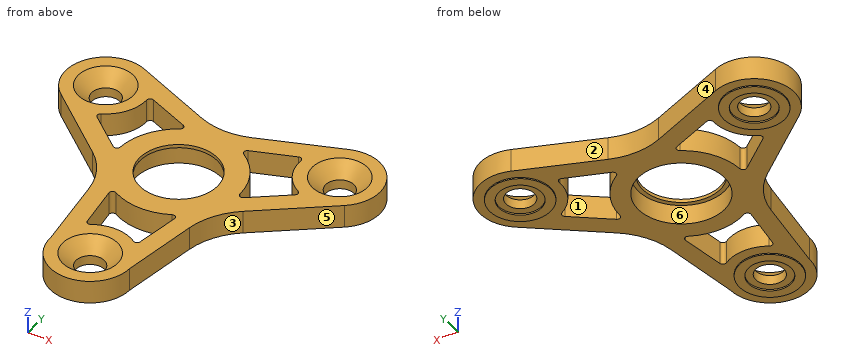
```python
from build123d import *

# Parameters (mm, degrees)
SKETCH_1_R          = 5.935
SKETCH_1_R_2        = 2.095
SKETCH_1_R_3        = 5.74
EXTRUDE_1_DEPTH     = 3.4
SKETCH_3_R          = 6.38
CUT_EXTRUDE_1_DEPTH = 2.9
SKETCH_4_R          = 4.5
EXTRUDE_3_DEPTH     = 0.56
SKETCH_6_R          = 3.15
CUT_EXTRUDE_2_DEPTH = 0.6
SKETCH_7_R          = 3.15
CUT_EXTRUDE_3_DEPTH = 0.6
SKETCH_8_R          = 3.15
CUT_EXTRUDE_4_DEPTH = 0.6
CUT_EXTRUDE_5_DEPTH = 10
SKETCH_13_R         = 4.5
SKETCH_13_R_2       = 3.15
CUT_EXTRUDE_6_DEPTH = 0.37
SKETCH_14_R         = 4.5
SKETCH_14_R_2       = 3.15
CUT_EXTRUDE_7_DEPTH = 0.37
SKETCH_15_R         = 4.5
SKETCH_15_R_2       = 3.15
CUT_EXTRUDE_8_DEPTH = 0.37


with BuildPart() as part:
    # 草图1 → 凸台-拉伸1 (new body)
    # profile 1 of 4: a face of its own
    with BuildSketch(Plane.XY):
        with Locations((-17.593306078, 10.1575)):
            Circle(SKETCH_1_R)
        with Locations((-17.593306078, 10.1575)):
            Circle(SKETCH_1_R_2, mode=Mode.SUBTRACT)
    # profile 2 of 4: a face of its own
    with BuildSketch(Plane.XY):
        with Locations((17.593306078, 10.1575)):
            Circle(SKETCH_1_R)
        with Locations((17.593306078, 10.1575)):
            Circle(SKETCH_1_R_2, mode=Mode.SUBTRACT)
    # profile 3 of 4: a face of its own
    with BuildSketch(Plane.XY):
        with BuildLine():
            Line((-3.823709102, 11.054508427), (-15.39430283, 15.670086481))
            ThreePointArc((-15.39430283, 15.670086481), (-12.680297362, 13.487150186), (-11.658306078, 10.1575))
            ThreePointArc((-11.658306078, 10.1575), (-15.021547784, 4.808641778), (-21.299513922, 5.521958132))
            Line((-21.299513922, 5.521958132), (-11.31029049, -2.464624515))
            ThreePointArc((-11.31029049, -2.464624515), (-8.793601867, -5.406520994), (-7.538053442, -9.068770941))
            Line((-7.538053442, -9.068770941), (-5.935, -20.315))
            ThreePointArc((-5.935, -20.315), (0, -14.38), (5.935, -20.315))
            Line((5.935, -20.315), (7.538053442, -9.068770941))
            ThreePointArc((7.538053442, -9.068770941), (8.793601867, -5.406520994), (11.31029049, -2.464624515))
            Line((11.31029049, -2.464624515), (21.299513922, 5.521958132))
            ThreePointArc((21.299513922, 5.521958132), (12.46358448, 7.172507316), (15.39430283, 15.670086481))
            Line((15.39430283, 15.670086481), (3.823709102, 11.054508427))
            ThreePointArc((3.823709102, 11.054508427), (0, 10.32), (-3.823709102, 11.054508427))
        make_face()
        Circle(SKETCH_1_R_3, mode=Mode.SUBTRACT)
    # profile 4 of 4: a face of its own
    with BuildSketch(Plane.XY):
        with Locations((0, -20.315)):
            Circle(SKETCH_1_R)
        with Locations((0, -20.315)):
            Circle(SKETCH_1_R_2, mode=Mode.SUBTRACT)
    extrude(amount=EXTRUDE_1_DEPTH)

    # 草图3 → 切除-拉伸1 (cut)
    with BuildSketch(Plane(origin=(0, 0, 0), x_dir=(-1, 0, 0), z_dir=(0, 0, -1))):
        Circle(SKETCH_3_R)
    extrude(amount=-CUT_EXTRUDE_1_DEPTH, mode=Mode.SUBTRACT)

    # 草图4 → 凸台-拉伸3 (add)
    with BuildSketch(Plane(origin=(0, 0, 0), x_dir=(-1, 0, 0), z_dir=(0, 0, -1))):
        with Locations(Location((0, -20.315, 0), (0, 0, 180))):
            Circle(SKETCH_4_R)
        with Locations(Location((17.593306078, 10.1575, 0), (0, 0, 180))):
            Circle(SKETCH_4_R)
        with Locations(Location((-17.593306078, 10.1575, 0), (0, 0, 180))):
            Circle(SKETCH_4_R)
    extrude(amount=EXTRUDE_3_DEPTH)

    # 草图6 → 切除-拉伸2 (cut)
    with BuildSketch(Plane(origin=(0, 0, -0.56), x_dir=(-1, 0, 0), z_dir=(0, 0, -1))):
        with Locations((0, -20.315)):
            Circle(SKETCH_6_R)
    extrude(amount=-CUT_EXTRUDE_2_DEPTH, mode=Mode.SUBTRACT)

    # 草图7 → 切除-拉伸3 (cut)
    with BuildSketch(Plane(origin=(0, 0, -0.56), x_dir=(-1, 0, 0), z_dir=(0, 0, -1))):
        with Locations((-17.593306078, 10.1575)):
            Circle(SKETCH_7_R)
    extrude(amount=-CUT_EXTRUDE_3_DEPTH, mode=Mode.SUBTRACT)

    # 草图8 → 切除-拉伸4 (cut)
    with BuildSketch(Plane(origin=(0, 0, -0.56), x_dir=(-1, 0, 0), z_dir=(0, 0, -1))):
        with Locations((17.593306078, 10.1575)):
            Circle(SKETCH_8_R)
    extrude(amount=-CUT_EXTRUDE_4_DEPTH, mode=Mode.SUBTRACT)

    # 草图9 → 切除-旋转1 (revolve, cut)
    with BuildSketch(Plane(origin=(0, 10.1575, 0), x_dir=(-1, 0, 0), z_dir=(0, -1, 0))):
        Polygon((19.688306078, -3.4), (19.688306078, -1.425), (21.663306078, -3.4), align=None)
    revolve(axis=Axis((-17.593306078, 10.1575, 3.4), (0, 0, -1)), mode=Mode.SUBTRACT)

    # 草图10 → 切除-旋转2 (revolve, cut)
    with BuildSketch(Plane(origin=(8.796653039, -5.07875, 0), x_dir=(0, 0, 1), z_dir=(-0.8660254037844397, 0.49999999999999806, 0)), mode=Mode.PRIVATE) as cut_revolve_2_sk:
        Polygon((3.4, 19.688306078), (3.4, 21.663306078), (1.425, 19.688306078), align=None)
    revolve(cut_revolve_2_sk.sketch.rotate(Axis((17.593306078, 10.1575, 3.4), (0, 0, -1)), 240), axis=Axis((17.593306078, 10.1575, 3.4), (0, 0, -1)), mode=Mode.SUBTRACT)

    # 草图11 → 切除-旋转3 (revolve, cut)
    with BuildSketch(Plane(origin=(8.796653039, -5.07875, 0), x_dir=(0, 0, 1), z_dir=(-0.8660254037844397, 0.49999999999999806, 0)), mode=Mode.PRIVATE) as cut_revolve_3_sk:
        Polygon((3.4, -15.498306078), (3.4, -13.523306078), (1.425, -15.498306078), align=None)
    revolve(cut_revolve_3_sk.sketch.rotate(Axis((0, -20.315, 3.4), (0, 0, -1)), 240), axis=Axis((0, -20.315, 3.4), (0, 0, -1)), mode=Mode.SUBTRACT)

    # 草图12 → 切除-拉伸5 (cut)
    with BuildSketch(Plane(origin=(0, 0, 0), x_dir=(-1, 0, 0), z_dir=(0, 0, -1))):
        with BuildLine():
            Line((9.80504906, -0.039344726), (14.886999287, 4.00948902))
            ThreePointArc((14.886999287, 4.00948902), (15.07318502, 4.447954395), (14.80758098, 4.843392767))
            ThreePointArc((14.80758098, 4.843392767), (12.397153655, 7.1575), (11.598291667, 10.402044914))
            ThreePointArc((11.598291667, 10.402044914), (11.388634011, 10.829783946), (10.915818991, 10.887775059))
            Line((10.915818991, 10.887775059), (4.868450998, 8.511093935))
            ThreePointArc((4.868450998, 8.511093935), (4.553503625, 8.092216181), (4.785479185, 7.622282399))
            ThreePointArc((4.785479185, 7.622282399), (7.794228634, 4.5), (8.993829785, 0.333205344))
            ThreePointArc((8.993829785, 0.333205344), (9.284816598, -0.102658275), (9.80504906, -0.039344726))
        make_face()
        with BuildLine():
            Line((3.971180296, -14.897264079), (4.936598062, -8.471749209))
            ThreePointArc((4.936598062, -8.471749209), (4.731312973, -7.989557906), (4.2083506, -7.955487743))
            ThreePointArc((4.2083506, -7.955487743), (0, -9), (-4.2083506, -7.955487743))
            ThreePointArc((-4.2083506, -7.955487743), (-4.731312973, -7.989557906), (-4.936598062, -8.471749209))
            Line((-4.936598062, -8.471749209), (-3.971180296, -14.897264079))
            ThreePointArc((-3.971180296, -14.897264079), (-3.684551009, -15.277738341), (-3.209289313, -15.245437681))
            ThreePointArc((-3.209289313, -15.245437681), (0, -14.315), (3.209289313, -15.245437681))
            ThreePointArc((3.209289313, -15.245437681), (3.684551009, -15.277738341), (3.971180296, -14.897264079))
        make_face()
        with BuildLine():
            Line((-4.868450998, 8.511093935), (-10.915818991, 10.887775059))
            ThreePointArc((-10.915818991, 10.887775059), (-11.388634011, 10.829783946), (-11.598291667, 10.402044914))
            ThreePointArc((-11.598291667, 10.402044914), (-11.594552605, 10.279797865), (-11.593306078, 10.1575))
            ThreePointArc((-11.593306078, 10.1575), (-12.459382111, 7.052210206), (-14.80758098, 4.843392767))
            ThreePointArc((-14.80758098, 4.843392767), (-15.07318502, 4.447954395), (-14.886999287, 4.00948902))
            Line((-14.886999287, 4.00948902), (-9.80504906, -0.039344726))
            ThreePointArc((-9.80504906, -0.039344726), (-9.284816598, -0.102658275), (-8.993829785, 0.333205344))
            ThreePointArc((-8.993829785, 0.333205344), (-7.794228634, 4.5), (-4.785479185, 7.622282399))
            ThreePointArc((-4.785479185, 7.622282399), (-4.553503625, 8.092216181), (-4.868450998, 8.511093935))
        make_face()
    extrude(amount=-CUT_EXTRUDE_5_DEPTH, mode=Mode.SUBTRACT)

    # 草图13 → 切除-拉伸6 (cut)
    with BuildSketch(Plane(origin=(0, 0, -0.56), x_dir=(-1, 0, 0), z_dir=(0, 0, -1))):
        with Locations(Location((0, -20.315, 0), (0, 0, 180))):
            Circle(SKETCH_13_R)
        with Locations((0, -20.315)):
            Circle(SKETCH_13_R_2, mode=Mode.SUBTRACT)
    extrude(amount=-CUT_EXTRUDE_6_DEPTH, mode=Mode.SUBTRACT)

    # 草图14 → 切除-拉伸7 (cut)
    with BuildSketch(Plane(origin=(0, 0, -0.56), x_dir=(-1, 0, 0), z_dir=(0, 0, -1))):
        with Locations(Location((-17.593306078, 10.1575, 0), (0, 0, 180))):
            Circle(SKETCH_14_R)
        with Locations((-17.593306078, 10.1575)):
            Circle(SKETCH_14_R_2, mode=Mode.SUBTRACT)
    extrude(amount=-CUT_EXTRUDE_7_DEPTH, mode=Mode.SUBTRACT)

    # 草图15 → 切除-拉伸8 (cut)
    with BuildSketch(Plane(origin=(0, 0, -0.56), x_dir=(-1, 0, 0), z_dir=(0, 0, -1))):
        with Locations(Location((17.593306078, 10.1575, 0), (0, 0, 180))):
            Circle(SKETCH_15_R)
        with Locations((17.593306078, 10.1575)):
            Circle(SKETCH_15_R_2, mode=Mode.SUBTRACT)
    extrude(amount=-CUT_EXTRUDE_8_DEPTH, mode=Mode.SUBTRACT)


solid = part.part
```
Build history of the part. All positions in model axes, mm. Face numbers are marked on the shaded views. A direction names the side the tool comes from. Coordinates: 2 decimals unless noted, no trailing zeros. Order: outer loops, then holes, each group sorted by start corner. A loop starts at its lowest first (then second) coordinate and runs counter-clockwise, first axis right, second up. Notation, with made-up numbers: M 5,-29.5 L 28,-29.5 A23 cw 28,-14.5 Z; hole C 86.25,12.25 d10. An arc over 180 degrees is marked long. One line per question, with ' | ' between items. Start each with the question number.
1. Cut at B-B (y = -13.5). Write the cut outline in (x, z).
2. Tool access for the marked faces 1, 2 and 3: list every direction of +Z, -Z, +X, -X, +Y, -Y with a clear straight run to the whole face (end or side of a thin tool).
3. Mould opens along Y. For the marked faces 4, 5 and 6 say: +Y half, -Y half, draft (parallel to the pull), parting line (faces both ways), or undercut.
4. Wall check: line 1 along X through (y, z) = (-8, 2.5); line 2 along Y through (x, z) = (-1, 1.55); line 3 along Y through (x, z) = (5, 0.3). Give the ranges that are in metal, low to high. Write a range as [from, to].
5. Flat gauge pins, fed straight in: P1, Ø10, axis at x = 10.5, y = -6.5, coming from the -Z side; P2, Ø5, axis at x = -16, y = 9, coming from the -Z side; P3, Ø2, axis at x = -12.5, z = 1.5, coming from the +Y side. Where does each tip first touch, or does it go through?
6. Cut at A-A (x = 0). Count the separate pieces of the cut face and the enclosed holes in it, plus the area to 3 significant figures.
7. Cut at C-C (y = -4). Write the cut outline in (x, z).
The answers:
1) outline: M -6.91,0 L -4.18,0 L -4.18,3.4 L -6.91,3.4 Z; M 4.18,0 L 6.91,0 L 6.91,3.4 L 4.18,3.4 Z
2) face 1: +Z, -Z | face 2: +Z, -Z, +Y | face 3: +Z, -Z, +X, -Y
3) face 4: +Y half | face 5: -Y half | face 6: undercut
4) line 1: x = [-7.75, -4.75], [-4.12, 4.12], [4.75, 7.75] | line 2: y = [-26.17, -22.3], [-18.33, -14.4], [-8.94, -6.3], [6.3, 10.37] | line 3: y = [-23.51, -3.96], [3.96, 7.48], [8.56, 11.52]
5) P1: stops at z = 0 | P2: stops at z = -0.19 | P3: stops at y = 14.91
6) separate pieces: 4 | enclosed holes: 0 | area: 45.8 mm2
7) outline: M -9.76,0 L -4.97,0 L -4.97,2.9 L -4.12,2.9 L -4.12,3.4 L -9.76,3.4 Z; M 4.12,2.9 L 4.97,2.9 L 4.97,0 L 9.76,0 L 9.76,3.4 L 4.12,3.4 Z
